```python
from build123d import *

# Parameters (mm, degrees)
BOSS_EXTRUDE2_DEPTH = 100
SKETCH3_W           = 11
SKETCH3_H           = 22
SKETCH4_R           = 1
CUT_EXTRUDE1_DEPTH  = 2
SKETCH5_R           = 1
CUT_EXTRUDE2_DEPTH  = 2
CIRPATTERN1_COUNT   = 4
SKETCH8_R           = 2.5
SKETCH8_W           = 20
SKETCH8_H           = 5
BOSS_EXTRUDE3_DEPTH = 10
SKETCH6_W           = 10
SKETCH6_H           = 190
BOSS_EXTRUDE4_DEPTH = 115
SKETCH10_W          = 10
SKETCH10_H          = 190
SKETCH11_R          = 1
CUT_EXTRUDE3_DEPTH  = 2
SKETCH12_R          = 75
CUT_EXTRUDE4_DEPTH  = 30


with BuildPart() as part:
    # Sketch1 → Boss-Extrude2 (new body)
    with BuildSketch(Plane(origin=(0, 0, 0), x_dir=(1, 0, 0), z_dir=(0, 1, 0))):
        with BuildLine():
            ThreePointArc((75, 0), (53.033008589, 53.033008589), (0, 75))
            Line((0, 75), (0, -75))
            ThreePointArc((0, -75), (53.033008589, -53.033008589), (75, 0))
        make_face()
    extrude(amount=BOSS_EXTRUDE2_DEPTH)

    # Sketch3 → Cut-Revolve3 (revolve, cut)
    with BuildSketch(Plane(origin=(0, 0, 0), x_dir=(-1, 0, 0), z_dir=(0, -1, 0))):
        with Locations((-59.5, 11)):
            Rectangle(SKETCH3_W, SKETCH3_H)
    cut_revolve3 = revolve(axis=Axis((0, 0, 0), (1, 0, 0)), mode=Mode.SUBTRACT)

    # Sketch4 → Cut-Extrude1 (cut)
    with BuildSketch(Plane.ZY.offset(-65)):
        Circle(SKETCH4_R)
    cut_extrude1 = extrude(amount=-CUT_EXTRUDE1_DEPTH, mode=Mode.SUBTRACT)

    # Sketch5 → Cut-Extrude2 (cut)
    with BuildSketch(Plane(origin=(54, 0, 0), x_dir=(0, 0, -1), z_dir=(1, 0, 0))):
        Circle(SKETCH5_R)
    cut_extrude2 = extrude(amount=-CUT_EXTRUDE2_DEPTH, mode=Mode.SUBTRACT)

    # CirPattern1: Cut-Revolve3, Cut-Extrude1, Cut-Extrude2 ×4 about axis
    cirpattern1_axis = Axis((0, 0, 0), (0, 1, 0))
    add([cut_revolve3.rotate(cirpattern1_axis, i * 360 / CIRPATTERN1_COUNT) for i in range(1, CIRPATTERN1_COUNT)], mode=Mode.SUBTRACT)
    add([cut_extrude1.rotate(cirpattern1_axis, i * 360 / CIRPATTERN1_COUNT) for i in range(1, CIRPATTERN1_COUNT)], mode=Mode.SUBTRACT)
    add([cut_extrude2.rotate(cirpattern1_axis, i * 360 / CIRPATTERN1_COUNT) for i in range(1, CIRPATTERN1_COUNT)], mode=Mode.SUBTRACT)

    # Sketch8 → Boss-Extrude3 (add)
    with BuildSketch(Plane.ZY):
        with Locations(Location((-70, 10, 0), (0, 0, 180))):
            Circle(SKETCH8_R)
        with Locations(Location((70, 10, 0), (0, 0, 180))):
            Circle(SKETCH8_R)
        with Locations((-30, 2.5)):
            Rectangle(SKETCH8_W, SKETCH8_H)
        with Locations((30, 2.5)):
            Rectangle(SKETCH8_W, SKETCH8_H)
    extrude(amount=BOSS_EXTRUDE3_DEPTH)

    # Sketch6 → Boss-Extrude4 (add)
    with BuildSketch(Plane(origin=(0, 100, 0), x_dir=(1, 0, 0), z_dir=(0, 1, 0))):
        with Locations((5, -95)):
            Rectangle(SKETCH6_W, SKETCH6_H)
    extrude(amount=BOSS_EXTRUDE4_DEPTH)

    # Sketch10 → Cut-Revolve4 (revolve, cut)
    with BuildSketch(Plane(origin=(0, 215, 0), x_dir=(1, 0, 0), z_dir=(0, 1, 0))):
        with Locations((5, -95)):
            Rectangle(SKETCH10_W, SKETCH10_H)
    revolve(axis=Axis((10, 215, 0), (-1, 0, 0)), mode=Mode.SUBTRACT)


with BuildPart() as cut_revolve4_kept_piece:
    # of the separate pieces the step leaves, the one the design keeps (cut_revolve4_pieces_kept)
    add(part.part.solids().sort_by_distance((0, 0, 75))[0])

    # Sketch11 → Cut-Extrude3 (cut)
    with BuildSketch(Plane.ZY.offset(-10)):
        with Locations((-0.669656263, 47.5)):
            Circle(SKETCH11_R)
        with Locations((-65.669656263, 60.5)):
            Circle(SKETCH11_R)
        with Locations((64.330343737, 60.5)):
            Circle(SKETCH11_R)
    extrude(amount=-CUT_EXTRUDE3_DEPTH, mode=Mode.SUBTRACT)

    # Sketch12 → Cut-Extrude4 (cut)
    with BuildSketch(Plane(origin=(0, 100, 0), x_dir=(1, 0, 0), z_dir=(0, 1, 0))):
        Circle(SKETCH12_R)
    extrude(amount=-CUT_EXTRUDE4_DEPTH, mode=Mode.SUBTRACT)


solid = cut_revolve4_kept_piece.part
```
Design review of the part built by this model. Coordinates are the model's own, in mm. A direction names the side the tool comes from. Coordinates: 2 decimals unless noted, no trailing zeros. Loops run counter-clockwise (first coordinate to the right, second up) from the corner with the lowest first, then second, coordinate; pieces in that order, holes last.
Q1. We need section C-C on y = 23.5. State the section outline as (x, z) points, and give its area (3 significant figures).
Reported:
outline: (0, -75) arc R75 ccw to (0, 75) - close
area: 8,840 mm2
Q2. We need section A-A on y = 16. State the section outline as (x, z) points.
Reported:
outline: (0, -75) arc R75 ccw to (0, 75) - (0, 65) - (15.1, 65) - (15.1, 54) - (0, 54) - (0, -54) - (15.1, -54) - (15.1, -65) - (0, -65) - close; hole (54, -15.1) - (65, -15.1) - (65, 15.1) - (54, 15.1) - close
Q3. To check wall thickness, follow line 1 (Z direction, x = 11, y = 60); line 2 (Y direction, x = 59, z = 0.5); line 3 (X direction, y = 37, z = 1.5) (3 decimals). State the ranges of each line that lie inside material, in increasing order.
Reported:
line 1: z = -74.19 to -66.54, -64.8 to 63.46, 65.2 to 74.19
line 2: y = 21.99 to 70
line 3: x = 10 to 74.985
Q4. We need section B-B on z = 16. State the section outline as (x, y) points.
Reported:
outline: (0, 0) - (54, 0) - (54, 15.1) - (65, 15.1) - (65, 0) - (73.27, 0) - (73.27, 70) - (10, 70) - (10, 25.67) - (0, 25.67) - close
Q5. Tool access review of faces 4 (the face through (-4.9, 11.5, -68)), 5 (the face through (8, 9, -54)), 6 (the face through (-5, 2, -20)), 7 (the face through (-5, 5, -30)): name each direction out of +Z, -Z, +X, -X, +Y, -Y from which nothing blocks a thin tool from reaching the whole face with its end or side.
Reported:
face 4: -X
face 5: -X, -Y
face 6: -X, +Y, -Y
face 7: +Z, -Z, -X, +Y
Q6. The part is to be moulded in two halves that separate along Z. For faces 1 (the face through (8, 9, -65)), 2 (the face through (-10, 10, 70)), 3 (the face through (74.98, 34.51, 1.65)), say which applies: +Z half, -Z half, draft (parallel to the pull), parting line (faces both ways), or undercut.
Reported:
face 1: undercut
face 2: draft
face 3: parting line
Q7. We need section D-D on z = 35.5. State the section outline as (x, y) points.
Reported:
outline: (-10, 0) - (66.07, 0) - (66.07, 70) - (10, 70) - (10, 28.35) - (0, 28.35) - (0, 5) - (-10, 5) - close
Q8. For pin 1 (3 mm diameter, centred on y = 10.5, z = -29.5, fed in from +X); pin 2 (1.8 mm diameter, centred on y = 60.5, z = -65.67, fed in from +X); pin 3 (0.6 mm diameter, centred on y = 61, z = -65.5, fed in from -X), all flat-tipped, find the tip position at first contact; note any pin that passes through.
Reported:
pin 1: stops at x = 69.58
pin 2: stops at x = 37.81
pin 3: stops at x = 12
